The listing builds one solid part. Answer for the finished solid, in the listing's coordinates (mm). A direction names the side the tool comes from. Coordinates: 2 decimals unless noted, no trailing zeros. Write each loop counter-clockwise with the first axis right and the second up, starting at its lowest first coordinate (ties: lowest second). Pieces come first, ordered by that corner, then holes.
Solid Edge part; units mm, degrees
sketch "Sketch1" plane through (0, 0, 0) normal (0, 0, 1) x (1, 0, 0)
  line L0 (50, -50) -> (50, 0)
  arc A0 (50, 0) -> (70.5719, -4.4281) centre (50, -50) cw
  arc A1 (70.5719, -4.4281) -> (50, 50) centre (0, 0) ccw
  arc A2 (-50, 50) -> (50, 50) centre (0, 0) cw
  arc A3 (-50, 50) -> (-70.5719, -4.4281) centre (0, 0) ccw
  arc A4 (-50, 0) -> (-70.5719, -4.4281) centre (-50, -50) ccw
  line L1 (-50, 0) -> (-50, -50)
  arc A5 (-50, -50) -> (50, -50) centre (0, 0) ccw
extrude "Protrusion1" add sketch "Sketch1" along normal blind 3
sketch "Sketch2" plane through (0, 0, 0) normal (0, 0, 1) x (1, 0, 0)
  circle A0 centre (-40.75, -34) radius 1
  circle A1 centre (40.75, -16) radius 1
  circle A2 centre (40.75, -34) radius 1
  circle A3 centre (-40.75, -16) radius 1
extrude "ExtrudedCutout_1" cut sketch "Sketch2" along normal blind 3
sketch "Sketch3" plane through (0, 0, 3) normal (0, 0, 1) x (0, 1, 0)
  circle A0 centre (11.2819, -60.2859) radius 1.5
  circle A1 centre (11.2819, 60.285) radius 1.5
  circle A2 centre (-60.3553, 0) radius 1.5
extrude "ExtrudedCutout_2" cut sketch "Sketch3" against normal blind 3
sketch "Sketch4" plane through (0, 0, 3) normal (0, 0, 1) x (0, 1, 0)
  circle A0 centre (-34, 40.75) radius 0.5
  circle A1 centre (-16, 40.75) radius 0.5
  circle A2 centre (-34, -40.75) radius 1.05
  circle A3 centre (-34, -40.75) radius 0.5
  circle A4 centre (-16, -40.75) radius 1
  circle A5 centre (-16, -40.75) radius 1.05
  circle A6 centre (-16, -40.75) radius 0.5
  circle A7 centre (-34, 40.75) radius 1.05
  circle A8 centre (-16, 40.75) radius 1.05
extrude "ExtrudedProtrusion_2" add sketch "Sketch4" along normal blind 142.4171
sketch "Sketch5" plane through (0, 0, 0) normal (0, 0, -1) x (0, 1, 0)
  circle A0 centre (-16, -40.75) radius 0.5
  circle A1 centre (-34, -40.75) radius 0.5
  circle A2 centre (-16, 40.75) radius 0.5
  circle A3 centre (-34, 40.75) radius 0.5
extrude "ExtrudedCutout_3" cut sketch "Sketch5" against normal blind 319.3791
sketch "Sketch6" plane through (0, 0, 3) normal (0, 0, 1) x (0, 1, 0)
  circle A0 centre (-16, 40.75) radius 1.05
  circle A1 centre (-34, 40.75) radius 1.05
  circle A2 centre (-16, -40.75) radius 1.05
  circle A3 centre (-34, -40.75) radius 1.05
extrude "ExtrudedCutout_4" cut sketch "Sketch6" along normal blind 870.2731
sketch "Sketch7" plane through (0, 0, 0) normal (0, 0, -1) x (0, 1, 0)
  circle A0 centre (-16, 40.75) radius 1.05
  circle A1 centre (-34, 40.75) radius 1.05
  circle A2 centre (-16, -40.75) radius 1.05
  circle A3 centre (-34, -40.75) radius 1.05
extrude "ExtrudedProtrusion_6" add sketch "Sketch7" against normal blind 0.5
sketch "Sketch8" plane through (40.75, -16, 0.5) normal (0, 0, 1) x (1, 0, 0)
  circle A0 centre (0, 0) radius 0.5
  circle A1 centre (0, -18) radius 0.5
  circle A2 centre (-81.5, 0) radius 0.5
  circle A3 centre (-81.5, -18) radius 0.5
extrude "Cutout1" cut sketch "Sketch8" against normal blind 3
1. Find the intervals of material crossed by L1, parallel to X at y = -16, z = 1.35; L2, parallel to Y at x = 40.75, z = 1.6; L3, parallel to Y at x = 40.75, z = 0.2, in increasing order.
Results found:
L1: x = -50 to -41.75, -39.75 to 39.75, 41.75 to 50
L2: y = -57.79 to -35, -33 to -17, -15 to 57.79
L3: y = -57.79 to -34.5, -33.5 to -16.5, -15.5 to 57.79
2. For a pull along X with two mould halves and no side action, classify faces 1 (the flat face through (-1, 1, 3)), 2 (the cylindrical face through (0.777, -70.706, 1.479)), 3 (the cylindrical face through (60.38, -1.09, 1.48)) as pulls with the +X half, pulls with the -X half, needs draft (parallel to the pull), parting line crosses it, or undercut.
Results found:
face 1: needs draft
face 2: parting line crosses it
face 3: undercut
3. Section A-A on z = 1 is taken. Give the vertices of the cut face in (x, y) (3 decimals), then the cut area to 3 significant figures.
Results found:
outline: (-70.572, -4.428) arc R50 cw to (-50, 0) - (-50, -50) arc R70.711 ccw to (50, -50) - (50, 0) arc R50 cw to (70.572, -4.428) arc R70.711 ccw (long way) to start; hole circle Ø3 at (-60.285, 11.282); hole circle Ø2 at (-40.75, -34); hole circle Ø2 at (-40.75, -16); hole circle Ø3 at (0, -60.355); hole circle Ø2 at (40.75, -34); hole circle Ø2 at (40.75, -16); hole circle Ø3 at (60.286, 11.282)
area: 14,300 mm2
4. Section B-B on y = 36.5 is taken. Give the vertices of the cut face in (x, z), then the cut area to 3 significant figures.
Results found:
outline: (-60.56, 0) - (60.56, 0) - (60.56, 3) - (-60.56, 3) - close
area: 363 mm2
5. Section C-C on y = -47 is taken. Give the vertices of the cut face in (x, z).
Results found:
outline: (-50, 0) - (50, 0) - (50, 3) - (-50, 3) - close
6. Flat-ended cylindrical pins translate along their axes: P1, Ø0.6, axis at x = -41, y = -34.5, coming from the +Z side; P2, Ø1, axis at x = 55.5, z = 2, coming from the -Y side; P3, Ø1, axis at y = 51.5, z = 1.5, coming from the +X side. Find the tip coordinate at first contact, or state that the pin passes through.
Results found:
P1: stops at z = 0.5
P2: stops at y = -0.36
P3: stops at x = 48.98
7. A tool of negligible diameter and unlimited length cuts with its end or side. For faces 4 (the cylindrical face through (-60.67, -1.15, 1.48)), 5 (the flat face through (-1, 1, 0)), from which of +Z, -Z, +X, -X, +Y, -Y can it reach the whole face along a straight path? Write none if from no direction.
Results found:
face 4: +Z, -Z, -Y
face 5: -Z, +X, -X, +Y, -Y
